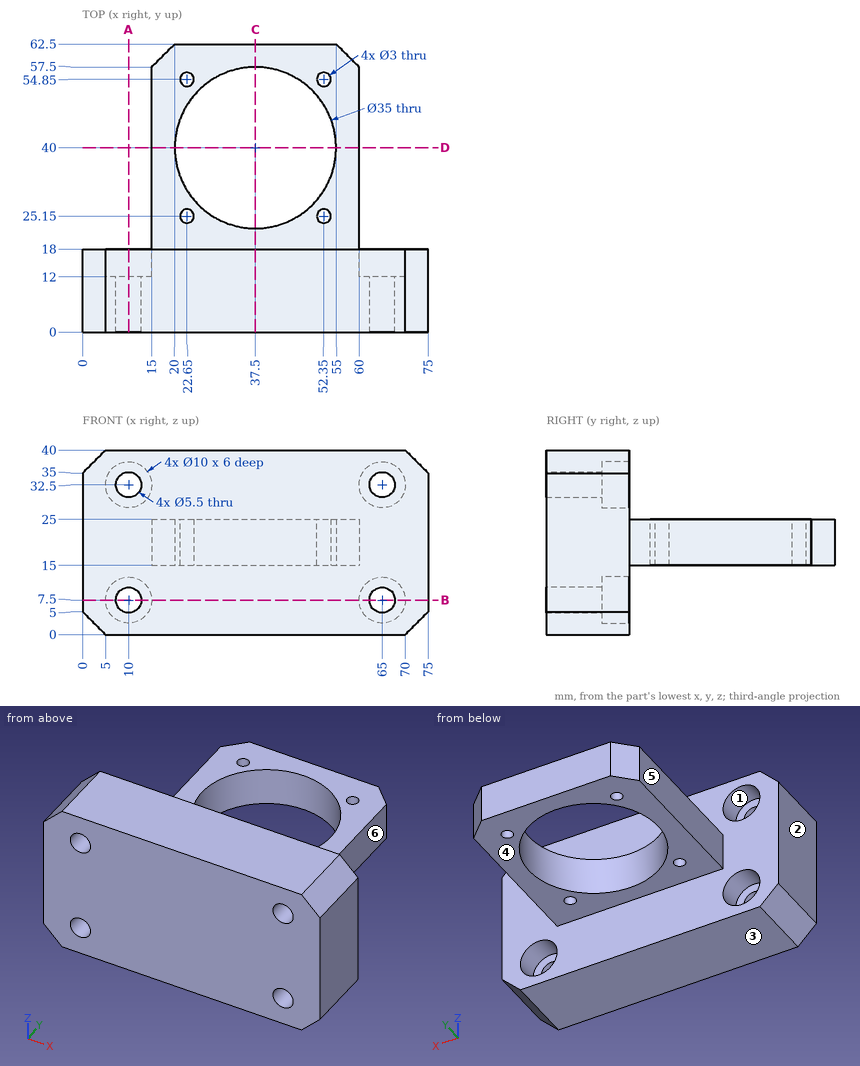
Drawing for the job (mm, zero at the part's lowest x, y, z). A direction names the side the tool comes from. Give positions to 0.01 mm unless a question says otherwise; leave off trailing zeros. Order: outer loops, then holes, each group sorted by start corner. A loop starts at its lowest first (then second) coordinate and runs counter-clockwise, first axis right, second up. Notation, with made-up numbers: (-19.75, 65.25) - (-3.75, 65.25) arc R24 cw to (-3.75, 94.25) - close; hole circle Ø11 at (26.5, 44.5). An arc over 180 degrees is marked (long way). Use one line per item in the form item = value.
Item 1: Probe probe 1 along X at (y, z) = (55, 24); probe 2 along Y at (x, z) = (52, 20); probe 3 along Z at (x, y) = (12.5, 15.5). List the from-to ranges inside material, lowest first. Write a range as from..to.
Solution:
probe_1 = 15..21.16, 24.14..28.49, 46.51..50.86, 53.84..60
probe_2 = 0..23.69, 26.61..30.2, 49.8..53.39, 56.31..62.5
probe_3 = 0..3.17, 11.83..28.17, 36.83..40
Item 2: Pin check, flat tips, straight feed: pin 1 Ø5 at (x, y) = (62.5, 11) entering from -Z; pin 2 Ø5 at (x, y) = (22.65, 25.15) entering from +Z; pin 3 Ø8 at (y, z) = (50, 18.5) entering from +X; pin 4 Ø6.5 at (x, z) = (10, 7.5) entering from +Y. Stop position of each tip, or through.
Solution:
pin_1 = 0
pin_2 = 25
pin_3 = 60
pin_4 = 12
Item 3: Which spindle directions (+Z, -Z, +X, -X, +Y, -Y) get a long thin tool onto all of the face, cutting with end or side? Do the marked faces 4, 5 and 6. Say none if no direction does.
Solution:
face_4 = -Z, +X, -X, +Y
face_5 = +Z, -Z, -X, +Y
face_6 = +Z, -Z, +X, +Y
Item 4: Two-plate mould, pull along X, no slides. Class the marked faces 1, 2 and 3: released by +X, released by -X, zero draft, split by the parting line, or undercut.
Solution:
face_1 = undercut
face_2 = released by -X
face_3 = zero draft
Item 5: Slice it at A-A on x = 10. Give the cut face in (y, z).
Solution:
outline = (0, 0) - (18, 0) - (18, 2.5) - (12, 2.5) - (12, 4.75) - (0, 4.75) - close; (0, 10.25) - (12, 10.25) - (12, 12.5) - (18, 12.5) - (18, 27.5) - (12, 27.5) - (12, 29.75) - (0, 29.75) - close; (0, 35.25) - (12, 35.25) - (12, 37.5) - (18, 37.5) - (18, 40) - (0, 40) - close
Item 6: Slice it at D-D on y = 40. Give the cut face in (x, z), and give its area (3 significant figures).
Solution:
outline = (15, 15) - (20, 15) - (20, 25) - (15, 25) - close; (55, 15) - (60, 15) - (60, 25) - (55, 25) - close
area = 100 mm2
Item 7: Slice it at B-B on z = 7.5. Give the cut face in (x, y).
Solution:
outline = (0, 0) - (7.25, 0) - (7.25, 12) - (5, 12) - (5, 18) - (0, 18) - close; (12.75, 0) - (62.25, 0) - (62.25, 12) - (60, 12) - (60, 18) - (15, 18) - (15, 12) - (12.75, 12) - close; (67.75, 0) - (75, 0) - (75, 18) - (70, 18) - (70, 12) - (67.75, 12) - close
Item 8: Slice it at C-C on x = 37.5. Give the cut face in (y, z).
Solution:
outline = (0, 0) - (18, 0) - (18, 15) - (22.5, 15) - (22.5, 25) - (18, 25) - (18, 40) - (0, 40) - close; (57.5, 15) - (62.5, 15) - (62.5, 25) - (57.5, 25) - close
